The model under review builds one solid part; all positions refer to its coordinate system, in mm. Face numbers are marked on the shaded views. A direction names the side the tool comes from. Give positions to 0.01 mm unless a question says otherwise; leave off trailing zeros. Write each loop counter-clockwise with the first axis right and the second up, starting at its lowest first coordinate (ties: lowest second). Pieces come first, ordered by that corner, then holes. Notation, with made-up numbers: (42.25, 62) - (72.25, 62) arc R12 cw to (72.25, 68) - close; hole circle Ø1 at (48, 10.5). An arc over 180 degrees is marked (long way). Write item = value, one per line.
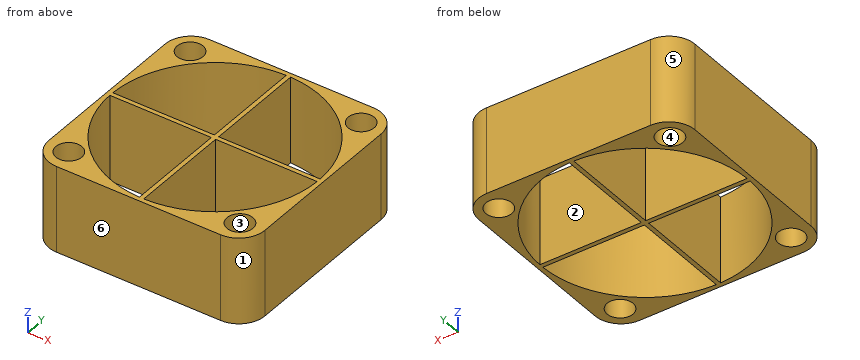
Autodesk Inventor part; units mm, degrees
ref_plane "YZ Plane" through (0, 0, 0) normal (1, 0, 0) x (0, 1, 0)
ref_plane "XZ Plane" through (0, 0, 0) normal (0, 1, 0) x (-1, 0, 0)
ref_plane "XY Plane" through (0, 0, 0) normal (0, 0, 1) x (1, 0, 0)
sketch "Sketch1" plane through (0, 0, 0) normal (0, 0, 1) x (1, 0, 0)
  line L0 (-12.5, -12.5) -> (12.5, -12.5)
  line L1 (12.5, -12.5) -> (12.5, 12.5)
  line L2 (12.5, 12.5) -> (-12.5, 12.5)
  line L3 (-12.5, 12.5) -> (-12.5, -12.5)
  line L4 (-12.5, -12.5) -> (12.5, 12.5) construction
  line L5 (12.5, -12.5) -> (-12.5, 12.5) construction
  point P0 (0, 0)
  dimension "d0" = 25
  dimension "d1" = 25
extrude "Extrusion1" add sketch "Sketch1" along normal blind 10
sketch "Sketch2" plane through (0, 0, 10) normal (0, 0, 1) x (1, 0, 0)
  circle A0 centre (0, 0) radius 14 construction
  line L0 (0, 0) -> (-9.8995, 9.8995) construction
  line L1 (-19.6, 0) -> (19.6, 0) construction
  line L2 (0, -19.6) -> (0, 19.6) construction
  point P0 (-9.8995, -9.8995)
  point P1 (9.8995, -9.8995)
  point P2 (9.8995, 9.8995)
  dimension "d4" = 28
  dimension "d5" = 45
  dimension "d8" = 360
hole "Hole1" at (-9.8995, 9.8995, 10) at (-9.8995, -9.8995, 10) at (9.8995, -9.8995, 10) at (9.8995, 9.8995, 10) direction (0, 0, -1) diameter 3 depth 15.25 tip angle 118
fillet "Fillet1" radius 3 4 edges at (-12.5, 12.5, 5) (12.5, 12.5, 5) (12.5, -12.5, 5) (-12.5, -12.5, 5)
sketch "Sketch3" plane through (0, 0, 10) normal (0, 0, 1) x (1, 0, 0)
  circle A0 centre (0, 0) radius 12
  dimension "d18" = 24
extrude "Extrusion2" cut sketch "Sketch3" against normal blind 10
sketch "Sketch4" plane through (0, 0, 10) normal (0, 0, 1) x (1, 0, 0)
  line L0 (-12.2062, -0.25) -> (12.2062, -0.25)
  line L1 (12.2062, -0.25) -> (12.2062, 0.25)
  line L2 (12.2062, 0.25) -> (-12.2062, 0.25)
  line L3 (-12.2062, 0.25) -> (-12.2062, -0.25)
  line L4 (-12.2062, -0.25) -> (12.2062, 0.25) construction
  line L5 (12.2062, -0.25) -> (-12.2062, 0.25) construction
  line L6 (-0.25, -12.2062) -> (0.25, -12.2062)
  line L7 (0.25, -12.2062) -> (0.25, 12.2062)
  line L8 (0.25, 12.2062) -> (-0.25, 12.2062)
  line L9 (-0.25, 12.2062) -> (-0.25, -12.2062)
  circle A0 centre (0, 0) radius 12
  line L10 (-0.25, -12.2062) -> (0.25, 12.2062) construction
  line L11 (0.25, -12.2062) -> (-0.25, 12.2062) construction
  dimension "d21" = 0.5
  dimension "d22" = 0.5
extrude "Extrusion3" add sketch "Sketch4" against normal blind 10 contours L3 L2 A0 L0 | A0 L2 L9 L0 | L9 L2 L7 L0 | L0 L7 A0 L9 | A0 L7 L6 L9 | L7 L2 A0 L0 | L9 A0 L7 L2 | L9 L8 L7 A0 | A0 L2 L1 L0
properties part number "Fan"
1. For line 1 (Y direction, x = 3.75, z = 4.25); line 2 (Y direction, x = 6.75, z = 4.25); line 3 (X direction, y = 2.75, z = 7.5), list the stretches that pass through material, from the lowest coordinate up. Write a range as from..to.
Findings below:
line_1 = -12.5..-11.4, -0.25..0.25, 11.4..12.5
line_2 = -12.5..-9.92, -0.25..0.25, 9.92..12.5
line_3 = -12.5..-11.68, -0.25..0.25, 11.68..12.5
2. Take a section at D-D on x = 10.25. Give the boundary of the cut face in (y, z), and give its area (3 significant figures).
Findings below:
outline = (-12.4, 0) - (-11.36, 0) - (-11.36, 10) - (-12.4, 10) - close; (-8.44, 0) - (-6.24, 0) - (-6.24, 10) - (-8.44, 10) - close; (-0.25, 0) - (0.25, 0) - (0.25, 10) - (-0.25, 10) - close; (6.24, 0) - (8.44, 0) - (8.44, 10) - (6.24, 10) - close; (11.36, 0) - (12.4, 0) - (12.4, 10) - (11.36, 10) - close
area = 70.0 mm²
3. Insertion check: P1, Ø3, axis at x = 2, y = -8.5, coming from the -Z side. The pin has a flat end and moves straight along its axis. Give the tip position at first contact, or say it passes through.
Findings below:
P1 = through
4. Take a section at B-B on x = -6.25. Give the boundary of the cut face in (y, z).
Findings below:
outline = (-12.5, 0) - (-10.24, 0) - (-10.24, 10) - (-12.5, 10) - close; (-0.25, 0) - (0.25, 0) - (0.25, 10) - (-0.25, 10) - close; (10.24, 0) - (12.5, 0) - (12.5, 10) - (10.24, 10) - close
5. Take a section at C-C on y = -4. Give the boundary of the cut face in (x, z).
Findings below:
outline = (-12.5, 0) - (-11.31, 0) - (-11.31, 10) - (-12.5, 10) - close; (-0.25, 0) - (0.25, 0) - (0.25, 10) - (-0.25, 10) - close; (11.31, 0) - (12.5, 0) - (12.5, 10) - (11.31, 10) - close
6. Machinability: for the marked faces 1 and 2, which of the approach directions +Z, -Z, +X, -X, +Y, -Y give a long, thin tool a straight path to every point of the face, cutting with its end or side? Answer none if there is none.
Findings below:
face_1 = +Z, -Z, +X, -Y
face_2 = +Z, -Z
7. Take a section at A-A on z = 3.5. Count the separate pieces of the cut face and the enclosed holes in it, and give its area (3 significant figures).
Findings below:
separate_pieces = 1
enclosed_holes = 8
area = 160 mm²
8. Draft analysis for pull direction Y (two halves, no side actions). For the marked faces 3, 4, 5 and 6, state which applies: +Y half, -Y half, draft (parallel to the pull), parting line (faces both ways), or undercut.
Findings below:
face_3 = undercut
face_4 = undercut
face_5 = +Y half
face_6 = -Y half
